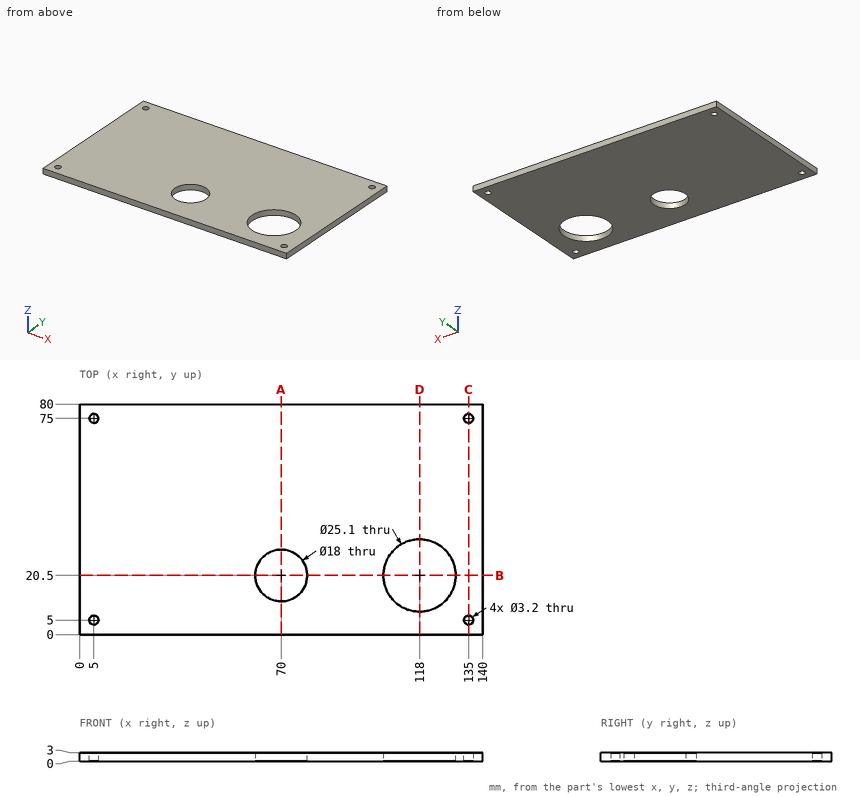
Drawing for the job (mm, zero at the part's lowest x, y, z). Give positions to 0.01 mm unless a question says otherwise; leave off trailing zeros. Loops run counter-clockwise (first coordinate to the right, second up) from the corner with the lowest first, then second, coordinate; pieces in that order, holes last. Notation, with made-up numbers: M 69.25,72 L 111.25,72 A21 cw 111.25,102 Z; hole C -7.75,21.5 d5. An arc over 180 degrees is marked long. Use one line per item in the form item = value.
Item 1: Flat gauge pin, fed straight in: pin 1 (22.5 mm diameter, centred on x = 118, y = 20.5, fed in from +Z). Where does the tip first touch, or does it go through?
Determined:
pin_1 = through
Item 2: Slice it at D-D (x = 118). List the corners of the cut face in (y, z).
Determined:
outline = M 0,0 L 7.95,0 L 7.95,3 L 0,3 Z; M 33.05,0 L 80,0 L 80,3 L 33.05,3 Z
Item 3: Slice it at B-B (y = 20.5). List the corners of the cut face in (x, z).
Determined:
outline = M 0,0 L 61,0 L 61,3 L 0,3 Z; M 79,0 L 105.45,0 L 105.45,3 L 79,3 Z; M 130.55,0 L 140,0 L 140,3 L 130.55,3 Z
Item 4: Slice it at A-A (x = 70). List the corners of the cut face in (y, z).
Determined:
outline = M 0,0 L 11.5,0 L 11.5,3 L 0,3 Z; M 29.5,0 L 80,0 L 80,3 L 29.5,3 Z
Item 5: Drill centre lines: probe 1 along Y at (x, z) = (5, 1); probe 2 along X at (y, z) = (20.5, 1.35); probe 3 along X at (y, z) = (5, 0.7). Where is each one in solid material? Low to high. Write a range as from..to.
Determined:
probe_1 = 0..3.4, 6.6..73.4, 76.6..80
probe_2 = 0..61, 79..105.45, 130.55..140
probe_3 = 0..3.4, 6.6..133.4, 136.6..140
Item 6: Slice it at C-C (x = 135). List the corners of the cut face in (y, z), plus the area to 3 significant figures.
Determined:
outline = M 0,0 L 3.4,0 L 3.4,3 L 0,3 Z; M 6.6,0 L 73.4,0 L 73.4,3 L 6.6,3 Z; M 76.6,0 L 80,0 L 80,3 L 76.6,3 Z
area = 221 mm2
